from build123d import *

# Parameters (mm, degrees)
SKETCH1_R           = 5
BOSS_EXTRUDE1_DEPTH = 17.5
SKETCH3_R           = 2.5
CUT_EXTRUDE1_DEPTH  = 16
SKETCH4_R           = 2.15
CUT_EXTRUDE2_DEPTH  = 26
SKETCH9_R           = 9.5
CUT_EXTRUDE5_DEPTH  = 1


with BuildPart() as part:
    # Sketch1 → Boss-Extrude1 (new, symmetric)
    with BuildSketch(Plane(origin=(0, 0, 0), x_dir=(0, 0, -1), z_dir=(1, 0, 0))):
        Polygon((-20, 26), (-7.85, 26), (-7.85, 25), (7.85, 25), (7.85, 26), (20, 26), (20, 18), (18, 16), (18, 5), (9.161099759, 5), (4.161099759, 0), (-4.161099759, 0), (-9.161099759, 5), (-18, 5), (-18, 16), (-20, 18), align=None)
        with Locations((0, 13)):
            Circle(SKETCH1_R, mode=Mode.SUBTRACT)
    extrude(amount=BOSS_EXTRUDE1_DEPTH, both=True)

    # Sketch3 → Cut-Extrude1 (cut)
    with BuildSketch(Plane(origin=(0, 18, 0), x_dir=(-1, 0, 0), z_dir=(0, 1, 0))):
        with Locations(Location((-10.5, 14, 0), (0, 0, 90))):
            Circle(SKETCH3_R)
        with Locations(Location((10.5, 14, 0), (0, 0, 90))):
            Circle(SKETCH3_R)
        with Locations(Location((-10.5, -14, 0), (0, 0, 90))):
            Circle(SKETCH3_R)
        with Locations(Location((10.5, -14, 0), (0, 0, 90))):
            Circle(SKETCH3_R)
    extrude(amount=CUT_EXTRUDE1_DEPTH, mode=Mode.SUBTRACT)

    # Sketch4 → Cut-Extrude2 (cut)
    with BuildSketch(Plane(origin=(0, 18, 0), x_dir=(-1, 0, 0), z_dir=(0, 1, 0))):
        with Locations(Location((-10.5, 14, 0), (0, 0, 90))):
            Circle(SKETCH4_R)
        with Locations(Location((10.5, 14, 0), (0, 0, 90))):
            Circle(SKETCH4_R)
        with Locations(Location((10.5, -14, 0), (0, 0, 90))):
            Circle(SKETCH4_R)
        with Locations(Location((-10.5, -14, 0), (0, 0, 90))):
            Circle(SKETCH4_R)
    extrude(amount=-CUT_EXTRUDE2_DEPTH, mode=Mode.SUBTRACT)

    # Sketch9 → Cut-Extrude5 (cut)
    with BuildSketch(Plane(origin=(17.5, 0, 0), x_dir=(0, 0, -1), z_dir=(1, 0, 0))):
        with Locations((0, 13)):
            Circle(SKETCH9_R)
    cut_extrude5 = extrude(amount=-CUT_EXTRUDE5_DEPTH, mode=Mode.SUBTRACT)

    # Mirror4: Cut-Extrude5 across plane
    add(cut_extrude5.mirror(Plane(origin=(0, 0, 0), x_dir=(0, 0, 1), z_dir=(1, 0, 0))), mode=Mode.SUBTRACT)


solid = part.part
CAD build for the part. Positions are in the model's coordinates, mm. A direction names the side the tool comes from. Coordinates: 2 decimals unless noted, no trailing zeros. Order: outer loops, then holes, each group sorted by start corner. A loop starts at its lowest first (then second) coordinate and runs counter-clockwise, first axis right, second up.
Item 1: Two-plate mould, pull along Z, no slides. Class faces 1 (the face through (0, 0, 0)), 2 (the face through (0, 22, -20)), 3 (the face through (9, 22, -16)): +Z half, -Z half, draft (parallel to the pull), parting line (faces both ways), or undercut.
Check sheet entries:
face 1: draft
face 2: -Z half
face 3: undercut
Item 2: Band-saw the part on D-D on z = 0. List the corners of the cut face in (x, y).
Check sheet entries:
outline: (-17.5, 0) - (17.5, 0) - (17.5, 3.5) - (16.5, 3.5) - (16.5, 8) - (-16.5, 8) - (-16.5, 3.5) - (-17.5, 3.5) - close; (-17.5, 22.5) - (-16.5, 22.5) - (-16.5, 18) - (16.5, 18) - (16.5, 22.5) - (17.5, 22.5) - (17.5, 25) - (-17.5, 25) - close
Item 3: 3-axis set-ups, long thin cutter, end or side, ignore diameter. For faces 4 (the face through (0, 10, 18)), 5 (the face through (-17.01, 21.01, -5.11)), 6 (the face through (0.2, 25.5, 7.85)), 7 (the face through (0, 5, -14)): which of +Z, -Z, +X, -X, +Y, -Y reach the whole face in a straight line?
Check sheet entries:
face 4: +Z, +X, -X, -Y
face 5: -X
face 6: +X, -X, +Y
face 7: -Z, +X, -X, -Y
Item 4: Band-saw the part on C-C on z = 14. List the corners of the cut face in (x, y), plus the area to 3 significant figures.
Check sheet entries:
outline: (-17.5, 5) - (-12.65, 5) - (-12.65, 18) - (-13, 18) - (-13, 26) - (-17.5, 26) - close; (-8.35, 5) - (8.35, 5) - (8.35, 18) - (8, 18) - (8, 26) - (-8, 26) - (-8, 18) - (-8.35, 18) - close; (12.65, 5) - (17.5, 5) - (17.5, 26) - (13, 26) - (13, 18) - (12.65, 18) - close
area: 543 mm2
Item 5: Pin check, flat tips, straight feed: pin 1 Ø4.5 at (x, z) = (-6.5, 14.5) entering from -Y; pin 2 Ø4 at (x, z) = (10.5, -14) entering from +Y; pin 3 Ø1 at (x, z) = (9.5, -4.5) entering from +Y; pin 4 Ø9 at (x, y) = (-6, 9) entering from -Z. Stop position of each tip, or through.
Check sheet entries:
pin 1: stops at y = 5
pin 2: passes through
pin 3: stops at y = 25
pin 4: stops at z = -18
Item 6: Band-saw the part on A-A on y = 13. List the corners of the cut face in (x, z).
Check sheet entries:
outline: (-17.5, -18) - (17.5, -18) - (17.5, -9.5) - (16.5, -9.5) - (16.5, -5) - (-16.5, -5) - (-16.5, -9.5) - (-17.5, -9.5) - close; (-17.5, 9.5) - (-16.5, 9.5) - (-16.5, 5) - (16.5, 5) - (16.5, 9.5) - (17.5, 9.5) - (17.5, 18) - (-17.5, 18) - close; hole circle Ø4.3 at (-10.5, -14); hole circle Ø4.3 at (-10.5, 14); hole circle Ø4.3 at (10.5, -14); hole circle Ø4.3 at (10.5, 14)
Item 7: Drill centre lines: L1, parallel to Z at x = 10.5, y = 23; L2, parallel to X at y = 13, z = -14; L3, parallel to Z at x = -12, y = 14.25. Where is each one in solid material? Low to high.
Check sheet entries:
L1: z = -20 to -16.5, -11.5 to 11.5, 16.5 to 20
L2: x = -17.5 to -12.65, -8.35 to 8.35, 12.65 to 17.5
L3: z = -18 to -15.54, -12.46 to -4.84, 4.84 to 12.46, 15.54 to 18
Item 8: Band-saw the part on B-B on x = -10.5. Give the number of separate pieces and of enclosed holes in the cut face, plus the area to 3 significant figures.
Check sheet entries:
separate pieces: 3
enclosed holes: 1
area: 573 mm2
